Source: CAD feature listing. Evaluate the final solid. Frame: model axes, mm. A direction names the side the tool comes from. Round coordinates to 2 decimals unless told otherwise and drop trailing zeros. Loops run counter-clockwise (first coordinate to the right, second up) from the corner with the lowest first, then second, coordinate; pieces in that order, holes last.
Item 1: Access query for faces 5 (the flat face through (-232.75, 3, -12)), 6 (the flat face through (-127, 3, -30)). Directions: +Z, -Z, +X, -X, +Y, -Y. A direction counts if a zero-diameter tool reaches every point of the face in a straight line with its end or side. Return the directions, or none.
Item 2: Pull-direction query (Z, two-part tool) for faces 1 (the flat face through (-244, 3, 0)), 2 (the flat face through (-231, 3, -7)), 3 (the flat face through (-11, 3, -7)), 4 (the flat face through (-17.25, 3, -3)); classes: released by +Z, released by -Z, zero draft, split by the parting line, or undercut.
Item 3: Ray query, L1, parallel to X at y = 0.3, z = -12; L2, parallel to X at y = 1.5, z = -6. Return the intervals inside material, ascending.
Item 4: First-contact query: P1, Ø2, axis at x = -14.5, y = 4, coming from the +Z side. Flat tip, straight axial feed; report the tip coordinate or a pass-through.
Item 5: Section query A-A on y = 2.35. Return loops of the section in (x, z).
Autodesk Inventor part; units mm, degrees
ref_plane "YZ Plane" through (0, 0, 0) normal (1, 0, 0) x (0, 1, 0)
ref_plane "XZ Plane" through (0, 0, 0) normal (0, 1, 0) x (-1, 0, 0)
ref_plane "XY Plane" through (0, 0, 0) normal (0, 0, 1) x (1, 0, 0)
sketch "Sketch3" plane through (0, 0, 0) normal (0, 1, 0) x (-1, 0, 0)
  line L0 (0, 0) -> (250, 0)
  line L1 (250, 0) -> (250, -30)
  line L2 (250, -30) -> (0, -30)
  line L3 (0, -30) -> (0, 0)
  dimension "d24" = 250
  dimension "d25" = 30
extrude "Extrusion2" add sketch "Sketch3" along normal blind 6
sketch "Sketch4" plane through (0, 6, 0) normal (0, 1, 0) x (1, 0, 0)
  line L0 (-250, 0) -> (0, 0)
  line L1 (-17.25, 0) -> (-12.75, 0)
  line L2 (-12.75, 0) -> (-12.75, 15)
  line L3 (-12.75, 15) -> (-17.25, 15)
  line L4 (-17.25, 15) -> (-17.25, 0)
  line L5 (-19, 5) -> (-11, 5)
  line L6 (-11, 5) -> (-11, 9)
  line L7 (-11, 9) -> (-19, 9)
  line L8 (-19, 9) -> (-19, 5)
  line L9 (0, 0) -> (0, 30)
  point P0 (-15, 9)
  point P1 (-15, 15)
  dimension "d28" = 4.5
  dimension "d29" = 15
  dimension "d30" = 8
  dimension "d31" = 5
  dimension "d32" = 4
  dimension "d33" = 12.75
extrude "Extrusion3" cut sketch "Sketch4" against normal through all
ref_plane "Work Plane13" through (-125, 0, 0) normal (1, 0, 0) x (0, 0, -1)
mirror "Mirror1" about plane through (-125, 0, 0) normal (1, 0, 0) of "Extrusion3"
properties part number "Selection_Ramp 1_Mid piece" material "Wood (Cherry)"
Data:
1. face 5: +Z, +Y, -Y
1. face 6: -Z, +X, -X, +Y, -Y
2. face 1: released by +Z
2. face 2: undercut
2. face 3: undercut
2. face 4: zero draft
3. L1: x = -250 to -237.25, -232.75 to -17.25, -12.75 to 0
3. L2: x = -250 to -239, -231 to -19, -11 to 0
4. P1: stops at z = -15
5. outline: (-250, -30) - (0, -30) - (0, 0) - (-12.75, 0) - (-12.75, -5) - (-11, -5) - (-11, -9) - (-12.75, -9) - (-12.75, -15) - (-17.25, -15) - (-17.25, -9) - (-19, -9) - (-19, -5) - (-17.25, -5) - (-17.25, 0) - (-232.75, 0) - (-232.75, -5) - (-231, -5) - (-231, -9) - (-232.75, -9) - (-232.75, -15) - (-237.25, -15) - (-237.25, -9) - (-239, -9) - (-239, -5) - (-237.25, -5) - (-237.25, 0) - (-250, 0) - close
